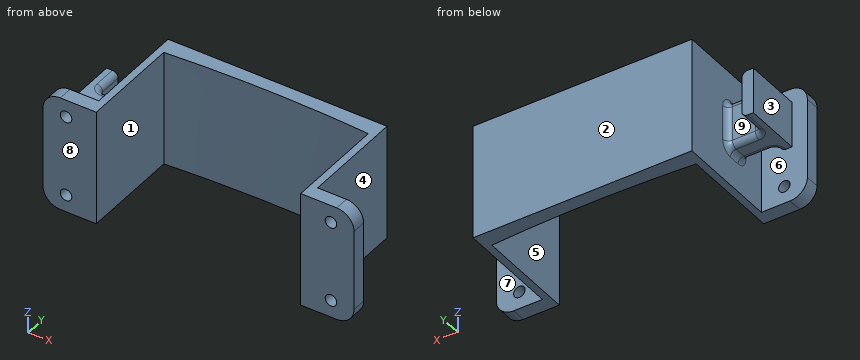
from build123d import *

# Parameters (mm, degrees)
BOSS_EXTRUDE1_DEPTH      = 20
SKETCH2_W                = 20
SKETCH2_H                = 2.5
BOSS_EXTRUDE2_DEPTH      = 8
SKETCH9_R                = 1
CORTE_EXTRUS_O1_DEPTH    = 39.118237105
FILETE1_R                = 3
ESBO_O8_W                = 0.75
ESBO_O8_H                = 17.5
CORTE_EXTRUS_O8_DEPTH    = 37.796738986
CORTE_EXTRUS_O9_DEPTH    = 37.796738986
FILETE1_OF_ESPELHAR1_R   = 3
ESBO_O14_W               = 8
ESBO_O14_H               = 4
RESSALTO_EXTRUS_O2_DEPTH = 6
ESBO_O15_W               = 8
ESBO_O15_H               = 10
RESSALTO_EXTRUS_O3_DEPTH = 2
FILETE3_R                = 1


with BuildPart() as part:
    # Sketch1 → Boss-Extrude1 (new body)
    with BuildSketch(Plane.XY):
        Polygon((17, -15), (19, -15), (19, 5.5), (-19, 5.5), (-19, -15), (-17, -15), (-17, 2.5), (17, 2.5), align=None)
    extrude(amount=BOSS_EXTRUDE1_DEPTH)

    # Sketch2 → Boss-Extrude2 (add)
    with BuildSketch(Plane(origin=(19, 0, 0), x_dir=(0, 0, -1), z_dir=(1, 0, 0))):
        with Locations((-10, -13.75)):
            Rectangle(SKETCH2_W, SKETCH2_H)
    boss_extrude2 = extrude(amount=BOSS_EXTRUDE2_DEPTH)

    # Sketch9 → Corte-extrusão1 (cut, through all)
    with BuildSketch(Plane(origin=(0, -12.5, 0), x_dir=(1, 0, 0), z_dir=(0, 1, 0))):
        with Locations(Location((23, -3, 0), (0, 0, 270))):
            Circle(SKETCH9_R)
        with Locations(Location((23, -17, 0), (0, 0, 270))):
            Circle(SKETCH9_R)
    corte_extrus_o1 = extrude(amount=-CORTE_EXTRUS_O1_DEPTH, mode=Mode.SUBTRACT)

    # Filete1
    filete1_edges = [part.edges().sort_by_distance(p)[0] for p in [
        (27, -13.75, 0),
        (27, -13.75, 20),
    ]]
    fillet(filete1_edges, radius=FILETE1_R)

    # Esboço8 → Corte-extrusão8 (cut, through all)
    with BuildSketch(Plane.XY.offset(20)):
        with Locations((17.375, -6.25)):
            Rectangle(ESBO_O8_W, ESBO_O8_H)
        with Locations((-17.375, -6.25)):
            Rectangle(ESBO_O8_W, ESBO_O8_H)
    extrude(amount=-CORTE_EXTRUS_O8_DEPTH, mode=Mode.SUBTRACT)

    # Esboço11 → Corte-extrusão9 (cut, through all)
    with BuildSketch(Plane.XY.offset(20)):
        with BuildLine():
            Line((-17.75, 2.5), (17.75, 2.5))
            add(Edge.make_bspline(
                [(-17.75, 2.5), (0, 3.750116691), (17.75, 2.5)],
                knots=[0, 0, 0, 1, 1, 1], degree=2))
        make_face()
    extrude(amount=-CORTE_EXTRUS_O9_DEPTH, mode=Mode.SUBTRACT)

    # Espelhar1: Boss-Extrude2, Corte-extrusão1 across plane
    add(boss_extrude2.mirror(Plane(origin=(0, 0, 0), x_dir=(0, 0, 1), z_dir=(1, 0, 0))))
    add(corte_extrus_o1.mirror(Plane(origin=(0, 0, 0), x_dir=(0, 0, 1), z_dir=(1, 0, 0))), mode=Mode.SUBTRACT)

    # Filete1 of Espelhar1
    filete1_of_espelhar1_edges = [part.edges().sort_by_distance(p)[0] for p in [
        (-27, -13.75, 0),
        (-27, -13.75, 20),
    ]]
    fillet(filete1_of_espelhar1_edges, radius=FILETE1_OF_ESPELHAR1_R)

    # Esboço14 → Ressalto-extrusão2 (add)
    with BuildSketch(Plane.ZY.offset(19)):
        with Locations((10, -5.5)):
            Rectangle(ESBO_O14_W, ESBO_O14_H)
    extrude(amount=RESSALTO_EXTRUS_O2_DEPTH)

    # Esboço15 → Ressalto-extrusão3 (add)
    with BuildSketch(Plane.ZY.offset(25)):
        with Locations((10, -3.5)):
            Rectangle(ESBO_O15_W, ESBO_O15_H)
    extrude(amount=RESSALTO_EXTRUS_O3_DEPTH)

    # Filete3
    filete3_edges = [part.edges().sort_by_distance(p)[0] for p in [
        (-19, -5.5, 6),
        (-22, -3.5, 6),
        (-19, -7.5, 10),
        (-22, -7.5, 6),
        (-19, -5.5, 14),
        (-22, -7.5, 14),
        (-19, -3.5, 10),
        (-22, -3.5, 14),
        (-25, -7.5, 10),
        (-25, -3.5, 10),
        (-25, -8, 14),
        (-25, -1, 14),
        (-25, -1, 6),
        (-25, -8, 6),
    ]]
    fillet(filete3_edges, radius=FILETE3_R - 0.0001)  # a hair under: the kernel refuses the full size


solid = part.part
Verification items for the finished model (mm, model axes). Face numbers are marked on the shaded views. A direction names the side the tool comes from. Give positions to 0.01 mm unless a question says otherwise; leave off trailing zeros. Write each loop counter-clockwise with the first axis right and the second up, starting at its lowest first coordinate (ties: lowest second). Pieces come first, ordered by that corner, then holes.
(1) Access from +Z, -Z, +X, -X, +Y, -Y to the whole of each face (thin tool, end or side, straight path). Record for the marked faces 5, 6, 7, 8 and 9.
(2) Mould release check, pull along X, two halves, no side actions. Record for the marked faces 1, 2, 3 and 4: +X half, -X half, draft (parallel to the pull), parting line (faces both ways), or undercut.
(3) Material ranges on line 1 (Z direction, x = -23, y = -14.1); line 2 (X direction, y = -14.4, z = 17); line 3 (X direction, y = -13.75, z = 14.25), recorded low to high.
(4) Cross-section at A-A (x = 23). Enter the section's corners in (y, z), plus the area to 3 significant figures.
(5) Cross-section at B-B (y = -5.25). Enter the section's corners in (x, z), plus the area to 3 significant figures.
(6) Gauge pin test, flat ends, axial feed: pin 1 (1 mm diameter, centred on x = -1, z = 6, fed in from -Y); pin 2 (0.6 mm diameter, centred on x = -26.5, z = 10, fed in from +Y); pin 3 (2.5 mm diameter, centred on x = -23.5, z = 12.5, fed in from +Y). Record the tip position at first contact, or that the pin passes through.
(7) Cross-section at D-D (y = -8). State how many separate pieces and enclosed holes the cut face has, plus the area to 3 significant figures.
(8) Cross-section at C-C (x = -22.5). Enter the section's corners in (y, z), plus the area to 3 significant figures.
Worked out:
1. face 5: +Z, -Z, -Y
1. face 6: +Z, -Z, -X
1. face 7: +Z, -Z, +X, +Y
1. face 8: +Z, -Z, +X, -X, -Y
1. face 9: +Z, -Z, +Y
2. face 1: undercut
2. face 2: draft
2. face 3: -X half
2. face 4: +X half
3. line 1: z = 0 to 2, 4 to 16, 18 to 20
3. line 2: x = -27 to -24, -22 to -17.75, 17.75 to 22, 24 to 27
3. line 3: x = -27 to -17.75, 17.75 to 27
4. outline: (-15, 0) - (-12.5, 0) - (-12.5, 2) - (-15, 2) - close; (-15, 4) - (-12.5, 4) - (-12.5, 16) - (-15, 16) - close; (-15, 18) - (-12.5, 18) - (-12.5, 20) - (-15, 20) - close
4. area: 40.0 mm2
5. outline: (-27, 6) - (-20, 6) arc R1 cw to (-19, 5) - (-19, 0) - (-17.75, 0) - (-17.75, 20) - (-19, 20) - (-19, 15) arc R1 cw to (-20, 14) - (-27, 14) - close; (17.75, 0) - (19, 0) - (19, 20) - (17.75, 20) - close
5. area: 114 mm2
6. pin 1: stops at y = 3.12
6. pin 2: stops at y = 1.5
6. pin 3: stops at y = -3.16
7. separate pieces: 3
7. enclosed holes: 0
7. area: 67.6 mm2
8. outline: (-15, 0) - (-12.5, 0) - (-12.5, 2.13) - (-15, 2.13) - close; (-15, 3.87) - (-12.5, 3.87) - (-12.5, 16.13) - (-15, 16.13) - close; (-15, 17.87) - (-12.5, 17.87) - (-12.5, 20) - (-15, 20) - close; (-7.5, 7) arc R1 ccw to (-6.5, 6) - (-4.5, 6) arc R1 ccw to (-3.5, 7) - (-3.5, 13) arc R1 ccw to (-4.5, 14) - (-6.5, 14) arc R1 ccw to (-7.5, 13) - close
8. area: 72.5 mm2
